Build history of the part. All positions in model axes, mm. A direction names the side the tool comes from. Coordinates: 2 decimals unless noted, no trailing zeros. Write each loop counter-clockwise with the first axis right and the second up, starting at its lowest first coordinate (ties: lowest second). Pieces come first, ordered by that corner, then holes.
Autodesk Inventor part; units mm, degrees
ref_plane "YZ Plane" through (0, 0, 0) normal (1, 0, 0) x (0, 1, 0)
ref_plane "XZ Plane" through (0, 0, 0) normal (0, 1, 0) x (-1, 0, 0)
ref_plane "XY Plane" through (0, 0, 0) normal (0, 0, 1) x (1, 0, 0)
sketch "Skizze1" plane through (0, 0, 0) normal (0, 0, 1) x (1, 0, 0)
  line L0 (-30, -17) -> (30, -17)
  line L1 (30, -17) -> (30, 17)
  line L2 (30, 17) -> (-30, 17)
  line L3 (-30, 17) -> (-30, -17)
  line L4 (-30, -17) -> (30, 17) construction
  line L5 (30, -17) -> (-30, 17) construction
  line L6 (-32, -19) -> (32, -19)
  line L7 (32, -19) -> (32, 19)
  line L8 (32, 19) -> (-32, 19)
  line L9 (-32, 19) -> (-32, -19)
  line L10 (-32, -19) -> (32, 19) construction
  line L11 (32, -19) -> (-32, 19) construction
  point P0 (0, 0)
  dimension "d0" = 38
  dimension "d1" = 64
  dimension "d2" = 2
  dimension "d3" = 2
extrude "Extrusion1" add sketch "Skizze1" along normal mid plane 30
sketch "Skizze2" plane through (-30, -17, -15) normal (1, 0, 0) x (0, 0, -1)
  circle A0 centre (-15, 17) radius 14
  dimension "d6" = 28
extrude "Extrusion2" add sketch "Skizze2" along normal up to next
sketch "Skizze3" plane through (32, -19, 15) normal (1, 0, 0) x (0, 0, -1)
  circle A0 centre (15, 19) radius 3
  dimension "d9" = 6
extrude "Extrusion3" cut sketch "Skizze3" against normal through all
sketch "Skizze4" plane through (-32, -19, 15) normal (-1, 0, 0) x (0, 0, 1)
  circle A0 centre (-15, 19) radius 8
  dimension "d12" = 16
extrude "Extrusion4" cut sketch "Skizze4" against normal blind 30
sketch "Skizze5" plane through (-32, 19, 15) normal (0, 1, 0) x (1, 0, 0)
  line L0 (19, 5) -> (47, 5)
  line L1 (47, 5) -> (47, 25)
  line L2 (47, 25) -> (19, 25)
  line L3 (19, 25) -> (19, 5)
  line L4 (19, 5) -> (47, 25) construction
  line L5 (47, 5) -> (19, 25) construction
  line L6 (64, 30) -> (64, 0)
  point P0 (32, 15)
  point P1 (33, 15)
  point P2 (33, 15)
  dimension "d15" = 28
  dimension "d16" = 20
  dimension "d17" = 17
hole "Bohrung1" at (-13, 19, -10) at (15, 19, -10) at (15, 19, 10) at (-13, 19, 10) direction (0, -1, 0) diameter 2.459 depth 2
sketch "Skizze6" plane through (-32, -19, 15) normal (0, -1, 0) x (1, 0, 0)
  circle A0 centre (47, -5) radius 1.2295
  circle A1 centre (19, -25) radius 1.2295
  circle A2 centre (47, -25) radius 1.2295
  circle A3 centre (19, -5) radius 1.2295
  line L0 (2, -30) -> (2, 0)
  line L1 (62, -30) -> (2, -30)
  line L2 (62, -30) -> (62, 0)
  line L3 (2, 0) -> (62, 0)
  point P0 (32, -15)
hole "Bohrung2" at (-13, -19, 10) at (-13, -19, -10) at (15, -19, -10) at (15, -19, 10) direction (0, 1, 0) diameter 2.459 depth 2
sketch "Skizze7" plane through (32, -19, 15) normal (1, 0, 0) x (0, 0, -1)
  circle A0 centre (-1, 20.5) radius 1
  circle A1 centre (-1, 17.5) radius 1
  line L0 (0, 0) -> (0, 38)
  line L1 (36.4, 19) -> (-8.4, 19)
  point P0 (15, 19)
  dimension "d32" = 2
  dimension "d34" = 3
  dimension "d35" = 1
extrude "Extrusion5" add sketch "Skizze7" along normal blind 5 and the other way blind 20
sketch "Skizze8" plane through (12, 1.5, 16) normal (-1, 0, 0) x (0, 0, 1)
  circle A0 centre (0, -3) radius 1
  circle A1 centre (0, 0) radius 1
  circle A2 centre (0, -3) radius 1
  circle A3 centre (0, 0) radius 1
  circle A4 centre (-16, -1.5) radius 14
  line L0 (-2.5175, -5.2711) -> (-2.5175, 7.0646)
  point P0 (-16, -1.5)
revolve "Umdrehung1" add sketch "Skizze8" angle 90 about axis through (12, -3.7711, 13.4825) along (0, -1, 0) contours A0 | A1
sketch "Skizze9" plane through (37, 1.5, 16) normal (1, 0, 0) x (0, 0, -1)
  circle A0 centre (0, 0) radius 1
sketch "Skizze10" plane through (37, -1.5, 16) normal (1, 0, 0) x (0, 0, -1)
  circle A0 centre (0, 0) radius 1
properties part number "Korper"
1. Saw through at D-D on y = -16. List the corners of the cut face in (x, z), plus the area to 3 significant figures.
Computed values:
outline: (-32, -15) - (-30, -15) - (-30, 15) - (-32, 15) - close; (30, -15) - (32, -15) - (32, 15) - (30, 15) - close
area: 120 mm2
2. Probe line 1 along Z through (x, y) = (15, 17.7); line 2 along Y through (x, z) = (-24, 0); line 3 along Y through (x, z) = (26.5, 1). List the from-to ranges inside material, lowest first.
Computed values:
line 1: z = -15 to -11.23, -8.77 to 8.77, 11.23 to 15
line 2: y = -19 to -17, -14 to -8, 8 to 14, 17 to 19
line 3: y = -19 to -17, -13.96 to -2.83, 2.83 to 13.96, 17 to 19
3. Saw through at A-A on x = -16. List the corners of the cut face in (y, z).
Computed values:
outline: (-19, -15) - (-17, -15) - (-17, 15) - (-19, 15) - close; circle Ø28 at (0, 0); (17, -15) - (19, -15) - (19, 15) - (17, 15) - close; hole circle Ø16 at (0, 0)
4. Flat gauge pins, fed straight in: pin 1 (1.5 mm diameter, centred on x = -13, z = 10, fed in from +Y); pin 2 (1.5 mm diameter, centred on y = 11, z = 2, fed in from +X); pin 3 (2 mm diameter, centred on x = 15, z = 10, fed in from -Y). Where does each tip first touch, or does it go through?
Computed values:
pin 1: stops at y = 10.51
pin 2: stops at x = 32
pin 3: stops at y = -10.72
5. 3-axis set-ups, long thin cutter, end or side, ignore diameter. For faces 5 (the face through (-17.21, -7.81, -1.73)), 6 (the face through (0, -17, 0)), 7 (the face through (13.963, -17.986, -10.661)), 8 (the face through (30, -4, -14)), 9 (the face through (-14.037, 17.986, -9.339)): which of +Z, -Z, +X, -X, +Y, -Y reach the whole face in a straight line?
Computed values:
face 5: -X
face 6: +Z, -Z
face 7: -Y
face 8: none
face 9: +Y
6. Saw through at C-C on z = 0. List the corners of the cut face in (x, y).
Computed values:
outline: (-32, -19) - (32, -19) - (32, -3) - (-2, -3) - (-2, -8) - (-32, -8) - close; (-32, 8) - (-2, 8) - (-2, 3) - (32, 3) - (32, 19) - (-32, 19) - close; hole (-30, -17) - (30, -17) - (30, -14) - (-30, -14) - close; hole (-30, 14) - (30, 14) - (30, 17) - (-30, 17) - close
7. Saw through at B-B on x = 26. List the corners of the cut face in (y, z), plus the area to 3 significant figures.
Computed values:
outline: (-19, -15) - (-17, -15) - (-17, 15) - (-19, 15) - close; circle Ø28 at (0, 0); circle Ø2 at (-1.5, 16); circle Ø2 at (1.5, 16); (17, -15) - (19, -15) - (19, 15) - (17, 15) - close; hole circle Ø6 at (0, 0)
area: 714 mm2
8. Mould opens along X. For faces 1 (the face through (-0.42, 5.362, -12.932)), 2 (the face through (0, -19, 0)), 3 (the face through (37, 2, 16)), 4 (the face through (-14.037, -17.986, -10.661)) say: +X half, -X half, draft (parallel to the pull), parting line (faces both ways), or undercut.
Computed values:
face 1: undercut
face 2: draft
face 3: +X half
face 4: undercut
